For this review, take the finished solid that the model builds, in its own axes (mm). A direction names the side the tool comes from. Coordinates: 2 decimals unless noted, no trailing zeros. Loops run counter-clockwise (first coordinate to the right, second up) from the corner with the lowest first, then second, coordinate; pieces in that order, holes last. Notation, with made-up numbers: M 9,33.5 L 30,33.5 A18 cw 30,60.5 Z; hole C 84.25,41 d7. An arc over 180 degrees is marked long. Answer as a JSON object with one key per item and string values. Group by question number.
Item 1: Add section D-D (z = -14). State the section outline as (x, y) points.
Item 2: Add section A-A (y = -2.25). State the section outline as (x, z) points.
Item 3: Add section B-B (x = -15). State the section outline as (y, z) points.
Item 4: Mouldability with a two-part tool opening along X and no side actions: class faces 1 (the face through (0, -10, 15)), 2 (the face through (-16.5, -2.46, -14.93)), 3 (the face through (-7.5, -10, 0)) as +X half, -X half, draft (parallel to the pull), parting line (faces both ways), or undercut.
Item 5: Wall thickness on L1, parallel to Z at x = 15, y = -3.65; L2, parallel to Z at x = 2, y = -8.5; L3, parallel to Y at x = -15, z = 6: over which ranges is each line inside the solid? List them lowest first. Write a range as from..to.
Item 6: Insertion check: pin 1 (1.5 mm diameter, centred on x = -5.5, z = 3.5, fed in from -Y); pin 2 (3 mm diameter, centred on y = -8.5, z = -15, fed in from +X); pin 3 (1.5 mm diameter, centred on x = -8, y = -12.5, fed in from +Z); pin 4 (2.5 mm diameter, centred on x = -15, z = 15, fed in from -Y). Each pin has a flat end and moves straight along its axis. Give the tip position at first contact, or say it passes through.
Item 7: Add section C-C (z = -3). State the section outline as (x, y) points, then the cut area to 3 significant figures.
Item 8: Tool access review of faces 4 (the face through (0, -2, -20)), 5 (the face through (0, -10, -15)), 6 (the face through (7.5, -10, 0)): name each direction out of +Z, -Z, +X, -X, +Y, -Y from which nothing blocks a thin tool from reaching the whole face with its end or side.
from build123d import *

# Parameters (mm, degrees)
F0_R     = 1.5
F1_DEPTH = 5
F3_DEPTH = 15
F4_R     = 5


with BuildPart() as f1:
    # F0 (on Front) → F1 (new body)
    with BuildSketch(Plane.XZ):
        with Locations((-15, -15)):
            Circle(F0_R)
        with BuildLine():
            ThreePointArc((16.5, -15), (15, -13.5), (13.5, -15))
            ThreePointArc((13.5, -15), (15, -16.5), (16.5, -15))
        make_face()
        Polygon((-20, 20), (-20, 0), (-20, -20), (20, -20), (20, 20), align=None)
        with Locations((-15, -15)):
            Circle(F0_R, mode=Mode.SUBTRACT)
        with BuildLine():
            ThreePointArc((16.5, -15), (15, -16.5), (13.5, -15))
            ThreePointArc((13.5, -15), (15, -13.5), (16.5, -15))
        make_face(mode=Mode.SUBTRACT)
        with Locations((-15, 15)):
            Circle(F0_R, mode=Mode.SUBTRACT)
        with Locations((15, 15)):
            Circle(F0_R, mode=Mode.SUBTRACT)
    extrude(amount=F1_DEPTH)

    # F2 (on face) → F3 (join)
    with BuildSketch(Plane.XZ.offset(5)):
        Polygon((7.5, 15), (0, 15), (-7.5, 15), (-7.5, -15), (7.5, -15), align=None)
    extrude(amount=F3_DEPTH)

    # F4
    f4_edges = [f1.edges().sort_by_distance(p)[0] for p in [
        (-7.5, -20, 0),
        (0, -20, 15),
        (7.5, -20, 0),
        (0, -20, -15),
    ]]
    fillet(f4_edges, radius=F4_R)


solid = f1.part
From the geometry:
{
 "1": {"outline": "M -20,-5 L -16.12,-5 L -16.12,0 L -20,0 Z; M -13.88,-5 L -7.5,-5 L -7.5,-15 A5 ccw -6.5,-18 L 6.5,-18 A5 ccw 7.5,-15 L 7.5,-5 L 13.88,-5 L 13.88,0 L -13.88,0 Z; M 16.12,-5 L 20,-5 L 20,0 L 16.12,0 Z"},
 "2": {"outline": "M -20,-20 L 20,-20 L 20,20 L -20,20 Z; hole C -15,-15 d3; hole C -15,15 d3; hole C 15,-15 d3; hole C 15,15 d3"},
 "3": {"outline": "M -5,-20 L 0,-20 L 0,-16.5 L -5,-16.5 Z; M -5,-13.5 L 0,-13.5 L 0,13.5 L -5,13.5 Z; M -5,16.5 L 0,16.5 L 0,20 L -5,20 Z"},
 "4": {"face 1": "draft", "face 2": "undercut", "face 3": "-X half"},
 "5": {"L1": "z = -20..-16.5, -13.5..13.5, 16.5..20", "L2": "z = -15..15", "L3": "y = -5..0"},
 "6": {"pin 1": "stops at y = -19.47", "pin 2": "stops at x = 7.5", "pin 3": "stops at z = 15", "pin 4": "passes through"},
 "7": {"outline": "M -20,-5 L -7.5,-5 L -7.5,-15 A5 ccw -2.5,-20 L 2.5,-20 A5 ccw 7.5,-15 L 7.5,-5 L 20,-5 L 20,0 L -20,0 Z", "area": "414 mm²"},
 "8": {"face 4": "-Z, +X, -X, +Y, -Y", "face 5": "-Z, +X, -X, -Y", "face 6": "+Z, -Z, +X, -Y"}
}
